Input: part model. Units: mm. Frame: model coordinates. Face numbers are marked on the shaded views. A direction names the side the tool comes from. Coordinates: 2 decimals unless noted, no trailing zeros. Write each loop counter-clockwise with the first axis right and the second up, starting at its lowest first coordinate (ties: lowest second). Pieces come first, ordered by that corner, then holes.
1) Section query D-D (z = -17.5). Output: boundary loops of the cut face in (x, y).
2) Section query A-A (z = -3.5). Output: boundary loops of the cut face in (x, y), then the cut area to 3 significant figures.
3) Section query B-B (x = 16.5). Output: boundary loops of the cut face in (y, z).
4) Pin query (flat end, axial travel): pin 1 Ø1.2 at (x, z) = (0.5, 10) entering from +Y; pin 2 Ø1.7 at (x, z) = (1, 1.5) entering from +Y; pin 3 Ø2 at (x, z) = (56, 6) entering from -Y. Return the tip coordinate at first contact, or that it passes through.
5) Draft query along Z for the marked faces 3, 4, 5 and 6. Return one class per face: pulls with the +Z half, pulls with the -Z half, needs draft (parallel to the pull), parting line crosses it, or undercut.
6) Line query: L1, parallel to Z at x = 53, y = 1; L2, parallel to X at y = -3.5, z = -8; L3, parallel to Y at x = 17, z = 23.5. Output: solid intervals per line, ascending.
7) Set-up query: the marked faces 1 and 2. Return all of +Z, -Z, +X, -X, +Y, -Y with unobstructed straight access to the full face (end or side cutting, diameter ignored); none if empty.
8) Section query C-C (y = -1.5). Output: boundary loops of the cut face in (x, z) (3 decimals).
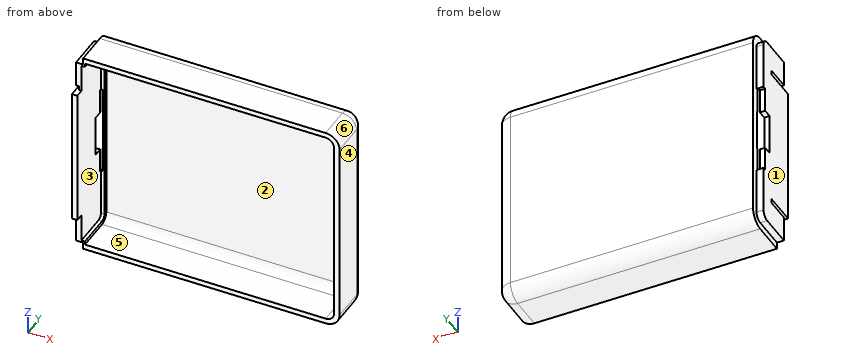
Autodesk Inventor part; units mm, degrees
ref_plane "YZ Plane" through (0, 0, 0) normal (1, 0, 0) x (0, 1, 0)
ref_plane "XZ Plane" through (0, 0, 0) normal (0, 1, 0) x (-1, 0, 0)
ref_plane "XY Plane" through (0, 0, 0) normal (0, 0, 1) x (1, 0, 0)
sketch "Sketch1" plane through (0, 0, 0) normal (1, 0, 0) x (0, 1, 0)
  line L0 (6.72, 30.5) -> (-6.72, 30.5)
  line L1 (-6.72, 30.5) -> (-6.72, -30.5)
  line L2 (-6.72, -30.5) -> (6.72, -30.5)
  line L3 (6.72, -30.5) -> (6.72, 30.5)
  line L4 (6.72, 0) -> (-6.72, 0) construction
  point P0 (0, 0)
  point P1 (0, 0)
  dimension "d0" = 61
  dimension "d1" = 13.44
extrude "Extrusion1" add sketch "Sketch1" along normal blind 75.6
sketch "Sketch2" plane through (0, -6.72, -30.5) normal (0, -1, 0) x (1, 0, 0)
  line L0 (1.54, 1.5) -> (74, 1.5)
  line L1 (74, 1.5) -> (74, 59.5)
  line L2 (74, 59.5) -> (1.54, 59.5)
  line L3 (1.54, 59.5) -> (1.54, 1.5)
  line L4 (0, 30.5) -> (1.54, 30.5) construction
  line L5 (0, 61) -> (0, 0) construction
  line L6 (75.6, 61) -> (75.6, 0) construction
  line L7 (0, 61) -> (75.6, 61) construction
  dimension "d4" = 1.54
  dimension "d5" = 1.6
  dimension "d6" = 1.5
extrude "Extrusion2" cut sketch "Sketch2" against normal blind 12.02
fillet "Fillet1" radius 4 5 edges at (37.8, 6.72, -30.5) (75.6, 6.72, 0) (75.6, 0, -30.5) (37.8, 6.72, 30.5) (75.6, 0, 30.5)
fillet "Fillet2" radius 2.4 5 edges at (74, -0.71, -29) (37.77, 5.3, -29) (74, 5.3, 0) (74, -0.71, 29) (37.77, 5.3, 29)
sketch "Sketch3" plane through (0, 0, 0) normal (-1, 0, 0) x (0, 0, 1)
  line L0 (-30.5, -6.72) -> (-30.5, 2.72)
  arc A0 (-26.5, 6.72) -> (-30.5, 2.72) centre (-26.5, 2.72) ccw
  line L1 (-26.5, 6.72) -> (26.5, 6.72)
  arc A1 (30.5, 2.72) -> (26.5, 6.72) centre (26.5, 2.72) ccw
  line L2 (30.5, 2.72) -> (30.5, -6.72)
  line L3 (28.55, -6.72) -> (28.55, 2.72)
  arc A2 (28.55, 2.72) -> (26.5, 4.77) centre (26.5, 2.72) ccw
  line L4 (26.5, 4.77) -> (-26.5, 4.77)
  arc A3 (-26.5, 4.77) -> (-28.55, 2.72) centre (-26.5, 2.72) ccw
  line L5 (-28.55, 2.72) -> (-28.55, -6.72)
  line L6 (-26.5, -6.72) -> (-30.5, -6.72) construction
  line L7 (-28.55, -6.72) -> (-30.5, -6.72)
  line L8 (28.55, -6.72) -> (30.5, -6.72)
  line L9 (-29, -6.72) -> (29, -6.72) construction
  point P0 (0, 0)
  dimension "d11" = 1.95
extrude "Extrusion3" cut sketch "Sketch3" against normal blind 2
sketch "Sketch4" plane through (1.54, -6.72, 28.55) normal (1, 0, 0) x (0, 0, -1)
  line L0 (1.95, 12.02) -> (55.15, 12.02)
  arc A0 (57.55, 9.62) -> (55.15, 12.02) centre (55.15, 9.62) ccw
  line L1 (57.55, 9.62) -> (57.55, 0)
  arc A1 (1.95, 12.02) -> (-0.45, 9.62) centre (1.95, 9.62) ccw
  line L2 (-0.45, 0) -> (-0.45, 9.62)
  line L3 (56.55, 0) -> (56.55, 9.62)
  arc A2 (56.55, 9.62) -> (55.15, 11.02) centre (55.15, 9.62) ccw
  line L4 (55.15, 11.02) -> (1.95, 11.02)
  arc A3 (1.95, 11.02) -> (0.55, 9.62) centre (1.95, 9.62) ccw
  line L5 (0.55, 9.62) -> (0.55, 0)
  line L6 (56.55, 0) -> (57.55, 0)
  line L7 (-0.45, 0) -> (0.55, 0)
  line L8 (57.1, 0) -> (0, 0) construction
  point P0 (28.55, 6.72)
  dimension "d14" = 1
extrude "Extrusion4" add sketch "Sketch4" along normal blind 1
sketch "Sketch5" plane through (0, 0, 0) normal (-1, 0, 0) x (0, 0, 1)
  arc A0 (-26.5, 6.72) -> (-30.5, 2.72) centre (-26.5, 2.72) ccw
  line L0 (-26.5, 6.72) -> (26.5, 6.72)
  line L1 (-30.5, -6.72) -> (-30.5, 2.72)
  line L2 (-29, -6.72) -> (-30.5, -6.72)
  line L3 (-28.55, -6.72) -> (-29, -6.72)
  line L4 (-28.55, 2.72) -> (-28.55, -6.72)
  arc A1 (-26.5, 4.77) -> (-28.55, 2.72) centre (-26.5, 2.72) ccw
  line L5 (26.5, 4.77) -> (-26.5, 4.77)
  arc A2 (30.5, 2.72) -> (26.5, 6.72) centre (26.5, 2.72) ccw
  arc A3 (28.55, 2.72) -> (26.5, 4.77) centre (26.5, 2.72) ccw
  line L6 (28.55, -6.72) -> (28.55, 2.72)
  line L7 (30.5, 2.72) -> (30.5, -6.72)
  line L8 (30.5, -6.72) -> (29, -6.72)
  line L9 (29, -6.72) -> (28.55, -6.72)
  point P0 (0, 0)
extrude "Extrusion5" cut sketch "Sketch5" against normal up to surface (2 mm away)
sketch "Sketch6" plane through (0, 0, 0) normal (-1, 0, 0) x (0, 0, 1)
  line L0 (26.5, 4.77) -> (-26.5, 4.77) construction
  line L1 (-13, 4.77) -> (13, 4.77)
  line L2 (13, 4.77) -> (13, 3.82)
  line L3 (13, 3.82) -> (-13, 3.82)
  line L4 (-13, 3.82) -> (-13, 4.77)
  line L5 (-26.5, 6.72) -> (26.5, 6.72) construction
  point P0 (0, 0)
  point P1 (0, 4.77)
  dimension "d19" = 26
  dimension "d21" = 2.9
extrude "Extrusion6" cut sketch "Sketch6" against normal up to surface (2 mm away)
sketch "Sketch7" plane through (0, 0, 0) normal (-1, 0, 0) x (0, 0, 1)
  line L0 (-5.925, 1.32) -> (5.925, 1.32)
  line L1 (5.925, 1.32) -> (5.925, 4.52)
  line L2 (5.925, 4.52) -> (-5.925, 4.52)
  line L3 (-5.925, 4.52) -> (-5.925, 1.32)
  line L4 (-26.5, 6.72) -> (26.5, 6.72) construction
  line L5 (0, 6.72) -> (0, 4.52) construction
  point P0 (0, 0)
  dimension "d24" = 2.2
  dimension "d25" = 3.2
  dimension "d26" = 11.85
extrude "Extrusion7" cut sketch "Sketch7" against normal up to surface (2.54 mm away)
sketch "Sketch8" plane through (0, 0, 0) normal (-1, 0, 0) x (0, 0, 1)
  line L0 (-19.935, -6.72) -> (19.935, -6.72)
  line L1 (19.935, -6.72) -> (19.935, -9.05)
  line L2 (19.935, -9.05) -> (-19.935, -9.05)
  line L3 (-19.935, -9.05) -> (-19.935, -6.72)
  line L4 (28.55, -6.72) -> (-28.55, -6.72) construction
  point P0 (0, 0)
  point P1 (0, -6.72)
  dimension "d29" = 39.87
  dimension "d30" = 2.33
extrude "Extrusion8" add sketch "Sketch8" against normal up to surface (1.54 mm away)
sketch "Sketch9" plane through (0, 0, 0) normal (-1, 0, 0) x (0, 0, 1)
  line L0 (-21.185, 0.16) -> (-19.935, 0.16)
  line L1 (-19.935, 0.16) -> (-19.935, -6.72)
  line L2 (-19.935, -6.72) -> (-21.185, -6.72)
  line L3 (-21.185, -6.72) -> (-21.185, 0.16)
  line L4 (19.935, 0.16) -> (21.185, 0.16)
  line L5 (21.185, 0.16) -> (21.185, -6.72)
  line L6 (21.185, -6.72) -> (19.935, -6.72)
  line L7 (19.935, -6.72) -> (19.935, 0.16)
  line L8 (-19.935, -3.28) -> (19.935, -3.28) construction
  line L9 (0, 0) -> (0, -3.28) construction
  line L10 (-19.935, -6.72) -> (-19.935, -9.05) construction
  line L11 (-19.935, -6.72) -> (-28.55, -6.72) construction
  dimension "d33" = 1.25
  dimension "d34" = 6.88
extrude "Extrusion9" cut sketch "Sketch9" against normal blind 0.85
properties part number "aus-200_top" material "PC/ABS Plastic"
Answer:
1. outline: (0, -9.05) - (1.54, -9.05) - (1.54, 4.3) - (2.54, 4.3) - (2.54, 5.3) - (71.6, 5.3) arc R2.4 cw to (74, 2.9) - (74, -6.72) - (75.6, -6.72) - (75.6, 2.72) arc R4 ccw to (71.6, 6.72) - (2, 6.72) - (2, 4.77) - (0, 4.77) - close
2. outline: (0, -9.05) - (1.54, -9.05) - (1.54, 1.32) - (0, 1.32) - close; (2, 4.52) - (2.54, 4.52) - (2.54, 5.3) - (71.6, 5.3) arc R2.4 cw to (74, 2.9) - (74, -6.72) - (75.6, -6.72) - (75.6, 2.72) arc R4 ccw to (71.6, 6.72) - (2, 6.72) - close
2. area: 138 mm2
3. outline: (-6.72, -30.5) - (2.72, -30.5) arc R4 ccw to (6.72, -26.5) - (6.72, 26.5) arc R4 ccw to (2.72, 30.5) - (-6.72, 30.5) - (-6.72, 29) - (2.9, 29) arc R2.4 cw to (5.3, 26.6) - (5.3, -26.6) arc R2.4 cw to (2.9, -29) - (-6.72, -29) - close
4. pin 1: stops at y = 3.82
4. pin 2: stops at y = 1.32
4. pin 3: stops at y = 5.3
5. face 3: undercut
5. face 4: needs draft
5. face 5: undercut
5. face 6: pulls with the +Z half
6. L1: z = -30.5 to -29, 29 to 30.5
6. L2: x = 0 to 1.54, 74 to 75.6
6. L3: y = 5.3 to 6.72
7. face 1: +Z, -Z, -X, +Y, -Y
7. face 2: -Y
8. outline: (0, -28.55) - (2, -28.55) - (2, -30.5) - (71.6, -30.5) arc R4 ccw to (75.6, -26.5) - (75.6, 26.5) arc R4 ccw to (71.6, 30.5) - (2, 30.5) - (2, 28.55) - (0, 28.55) - (0, 21.185) - (0.85, 21.185) - (0.85, 19.935) - (0, 19.935) - (0, -19.935) - (0.85, -19.935) - (0.85, -21.185) - (0, -21.185) - close; hole (1.54, -28) - (2.54, -28) - (2.54, -29) - (71.6, -29) arc R2.4 ccw to (74, -26.6) - (74, 26.6) arc R2.4 ccw to (71.6, 29) - (2.54, 29) - (2.54, 28) - (1.54, 28) - close
